from build123d import *

# Parameters (mm, degrees)
SKETCH1_W           = 304.8
SKETCH1_H           = 114.3
BOSS_EXTRUDE1_DEPTH = 12.7
SKETCH2_W           = 12.7
SKETCH2_H           = 114.3
CUT_EXTRUDE1_DEPTH  = 6.35
SKETCH3_W           = 114.3
SKETCH3_H           = 76.2
CUT_EXTRUDE2_DEPTH  = 6.35
CUT_EXTRUDE3_DEPTH  = 326.58847108


with BuildPart() as part:
    # Sketch1 → Boss-Extrude1 (new body)
    with BuildSketch(Plane(origin=(0, 0, 0), x_dir=(0, 0, -1), z_dir=(1, 0, 0))):
        with Locations((152.4, 57.15)):
            Rectangle(SKETCH1_W, SKETCH1_H)
    extrude(amount=BOSS_EXTRUDE1_DEPTH)

    # Sketch2 → Cut-Extrude1 (cut)
    with BuildSketch(Plane(origin=(12.7, 0, 0), x_dir=(0, 0, -1), z_dir=(1, 0, 0))):
        with Locations((6.35, 57.15)):
            Rectangle(SKETCH2_W, SKETCH2_H)
        with Locations((298.45, 57.15)):
            Rectangle(SKETCH2_W, SKETCH2_H)
        with Locations((133.35, 57.15)):
            Rectangle(SKETCH2_W, SKETCH2_H)
    extrude(amount=-CUT_EXTRUDE1_DEPTH, mode=Mode.SUBTRACT)

    # Sketch3 → Cut-Extrude2 (cut)
    with BuildSketch(Plane(origin=(12.7, 0, 0), x_dir=(0, 0, -1), z_dir=(1, 0, 0))):
        with Locations((69.85, 44.45)):
            Rectangle(SKETCH3_W, SKETCH3_H)
    extrude(amount=-CUT_EXTRUDE2_DEPTH, mode=Mode.SUBTRACT)

    # Sketch4 → Cut-Extrude3 (cut, through all)
    with BuildSketch(Plane(origin=(6.35, 0, 0), x_dir=(0, 0, -1), z_dir=(1, 0, 0))):
        with BuildLine():
            Line((19.05, 69.85), (19.05, 19.05))
            ThreePointArc((19.05, 19.05), (20.909871939, 14.559871939), (25.4, 12.7))
            Line((25.4, 12.7), (114.3, 12.7))
            ThreePointArc((114.3, 12.7), (118.790128061, 14.559871939), (120.65, 19.05))
            Line((120.65, 19.05), (120.65, 69.85))
            ThreePointArc((120.65, 69.85), (118.790128061, 74.340128061), (114.3, 76.2))
            Line((114.3, 76.2), (25.4, 76.2))
            ThreePointArc((25.4, 76.2), (20.909871939, 74.340128061), (19.05, 69.85))
        make_face()
    extrude(amount=-CUT_EXTRUDE3_DEPTH, mode=Mode.SUBTRACT)


solid = part.part
CAD build for the part. Positions are in the model's coordinates, mm. A direction names the side the tool comes from. Give positions to 0.01 mm unless a question says otherwise; leave off trailing zeros. Loops run counter-clockwise (first coordinate to the right, second up) from the corner with the lowest first, then second, coordinate; pieces in that order, holes last. Notation, with made-up numbers: M 65.5,-6 L 109.5,-6 A28 ccw 109.5,20 Z; hole C 45,-4 d5. An arc over 180 degrees is marked long. Write each question's results on one line, items separated by ' | '.
Q1. Probe probe 1 along Y at (x, z) = (7.5, -46); probe 2 along Z at (x, y) = (8.5, 93); probe 3 along Z at (x, y) = (6, 39). List the from-to ranges inside material, lowest first.
Geometry check:
probe 1: y = 0 to 6.35, 82.55 to 114.3 | probe 2: z = -292.1 to -139.7, -127 to -12.7 | probe 3: z = -304.8 to -120.65, -19.05 to 0
Q2. Band-saw the part on A-A on y = 63. Write the cut outline in (x, z).
Geometry check:
outline: M 0,-304.8 L 6.35,-304.8 L 6.35,-292.1 L 12.7,-292.1 L 12.7,-139.7 L 6.35,-139.7 L 6.35,-120.65 L 0,-120.65 Z; M 0,-19.05 L 6.35,-19.05 L 6.35,0 L 0,0 Z
Q3. Band-saw the part on D-D on y = 98. Write the cut outline in (x, z), and give its area (3 significant figures).
Geometry check:
outline: M 0,-304.8 L 6.35,-304.8 L 6.35,-292.1 L 12.7,-292.1 L 12.7,-139.7 L 6.35,-139.7 L 6.35,-127 L 12.7,-127 L 12.7,-12.7 L 6.35,-12.7 L 6.35,0 L 0,0 Z | area: 3,630 mm²
Q4. Which spindle directions (+Z, -Z, +X, -X, +Y, -Y) get a long thin tool onto all of the face, cutting with end or side? Do faces 4 (the face through (10, 82.55, -69)), 5 (the face through (10, 98, -12.7)), 6 (the face through (3.22, 74.29, -118.84)), 7 (the face through (10, 56, -292.1)), 8 (the face through (10, 3, -127)). Say none if no direction does.
Geometry check:
face 4: +Z, +X | face 5: +Z, +X, +Y, -Y | face 6: +X, -X | face 7: -Z, +X, +Y, -Y | face 8: +X, +Y, -Y
Q5. Mould opens along Y. For faces 1 (the face through (6, 0, -150)), 2 (the face through (10, 98, -127)), 3 (the face through (3, 12.7, -69)) say: pulls with the +Y half, pulls with the -Y half, needs draft (parallel to the pull), parting line crosses it, or undercut.
Geometry check:
face 1: pulls with the -Y half | face 2: needs draft | face 3: undercut
Q6. Flat gauge pins, fed straight in: P1, Ø5, axis at x = 8, y = 98, coming from the +Z side; P2, Ø5, axis at x = 9.5, y = 2.5, coming from the +Z side; P3, Ø10, axis at y = 63.5, z = -299, coming from the +X side; P4, Ø3, axis at x = 10.5, y = 3, coming from the -Z side. Where does each tip first touch, or does it go through?
Geometry check:
P1: stops at z = 0 | P2: stops at z = -12.7 | P3: stops at x = 6.35 | P4: stops at z = -292.1
Q7. Band-saw the part on C-C on z = -89.5. Write the cut outline in (x, y), and give its area (3 significant figures).
Geometry check:
outline: M 0,0 L 12.7,0 L 12.7,6.35 L 6.35,6.35 L 6.35,12.7 L 0,12.7 Z; M 0,76.2 L 6.35,76.2 L 6.35,82.55 L 12.7,82.55 L 12.7,114.3 L 0,114.3 Z | area: 565 mm²
Q8. Band-saw the part on B-B on x = 3.25. Write the cut outline in (y, z).
Geometry check:
outline: M 0,-304.8 L 114.3,-304.8 L 114.3,0 L 0,0 Z; hole M 12.7,-114.3 A6.35 ccw 19.05,-120.65 L 69.85,-120.65 A6.35 ccw 76.2,-114.3 L 76.2,-25.4 A6.35 ccw 69.85,-19.05 L 19.05,-19.05 A6.35 ccw 12.7,-25.4 Z
